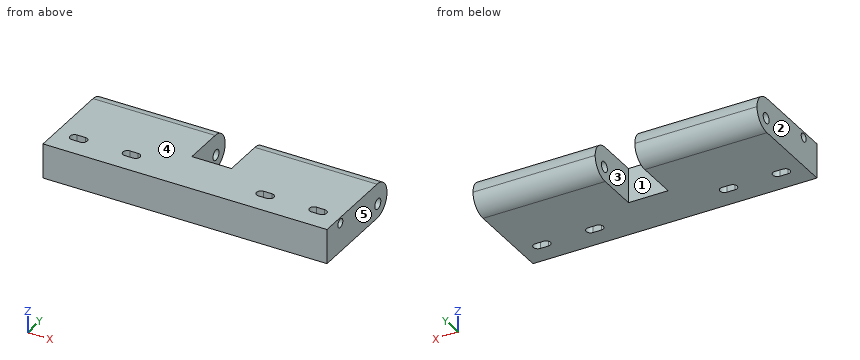
from build123d import *

# Parameters (mm, degrees)
SKETCH_1_W          = 172.02
SKETCH_1_H          = 28
EXTRUDE_1_DEPTH     = 21
SKETCH_2_W          = 74
SKETCH_2_H          = 21
EXTRUDE_2_DEPTH     = 35
CUT_EXTRUDE_1_DEPTH = 173.02
SKETCH_4_R          = 3.15
CUT_EXTRUDE_2_DEPTH = 173.02
SKETCH_6_R          = 2.6
CUT_EXTRUDE_3_DEPTH = 8
SKETCH_7_R          = 2.6
CUT_EXTRUDE_4_DEPTH = 8


with BuildPart() as part:
    # 草图1 → 凸台-拉伸1 (new body)
    with BuildSketch(Plane.XY):
        Rectangle(SKETCH_1_W, SKETCH_1_H)
        with BuildLine():
            Line((75.01, -2.7), (70.01, -2.7))
            ThreePointArc((70.01, -2.7), (67.31, 0), (70.01, 2.7))
            Line((70.01, 2.7), (75.01, 2.7))
            ThreePointArc((75.01, 2.7), (77.71, 0), (75.01, -2.7))
        make_face(mode=Mode.SUBTRACT)
        with BuildLine():
            Line((43.01, -2.7), (38.01, -2.7))
            ThreePointArc((38.01, -2.7), (35.31, 0), (38.01, 2.7))
            Line((38.01, 2.7), (43.01, 2.7))
            ThreePointArc((43.01, 2.7), (45.71, 0), (43.01, -2.7))
        make_face(mode=Mode.SUBTRACT)
        with BuildLine():
            Line((-70.01, -2.7), (-75.01, -2.7))
            ThreePointArc((-75.01, -2.7), (-77.71, 0), (-75.01, 2.7))
            Line((-75.01, 2.7), (-70.01, 2.7))
            ThreePointArc((-70.01, 2.7), (-67.31, 0), (-70.01, -2.7))
        make_face(mode=Mode.SUBTRACT)
        with BuildLine():
            Line((-43.01, 2.7), (-38.01, 2.7))
            ThreePointArc((-38.01, 2.7), (-35.31, 0), (-38.01, -2.7))
            Line((-38.01, -2.7), (-43.01, -2.7))
            ThreePointArc((-43.01, -2.7), (-45.71, 0), (-43.01, 2.7))
        make_face(mode=Mode.SUBTRACT)
    extrude(amount=EXTRUDE_1_DEPTH)

    # 草图2 → 凸台-拉伸2 (add)
    with BuildSketch(Plane(origin=(0, 14, 0), x_dir=(1, 0, 0), z_dir=(0, 1, 0))):
        with Locations((-49.01, -10.5)):
            Rectangle(SKETCH_2_W, SKETCH_2_H)
        with Locations((49.01, -10.5)):
            Rectangle(SKETCH_2_W, SKETCH_2_H)
    extrude(amount=EXTRUDE_2_DEPTH)

    # 草图3 → 切除-拉伸1 (cut, through all)
    with BuildSketch(Plane(origin=(86.01, 0, 0), x_dir=(0, 0, -1), z_dir=(1, 0, 0))):
        with BuildLine():
            Line((0, 49), (-10.5, 49))
            ThreePointArc((-10.5, 49), (-3.075378798, 45.924621202), (0, 38.5))
            Line((0, 38.5), (0, 49))
        make_face()
        with BuildLine():
            Line((-10.5, 49), (-21, 49))
            Line((-21, 49), (-21, 38.5))
            ThreePointArc((-21, 38.5), (-17.924621202, 45.924621202), (-10.5, 49))
        make_face()
    extrude(amount=-CUT_EXTRUDE_1_DEPTH, mode=Mode.SUBTRACT)

    # 草图4 → 切除-拉伸2 (cut, through all)
    with BuildSketch(Plane(origin=(86.01, 0, 0), x_dir=(0, 0, -1), z_dir=(1, 0, 0))):
        with Locations((-8.500165561, 39.35)):
            Circle(SKETCH_4_R)
    extrude(amount=-CUT_EXTRUDE_2_DEPTH, mode=Mode.SUBTRACT)

    # 草图6 → 切除-拉伸3 (cut)
    with BuildSketch(Plane(origin=(86.01, 0, 0), x_dir=(0, 0, -1), z_dir=(1, 0, 0))):
        with Locations((-17.5, 0)):
            Circle(SKETCH_6_R)
    extrude(amount=-CUT_EXTRUDE_3_DEPTH, mode=Mode.SUBTRACT)

    # 草图7 → 切除-拉伸4 (cut)
    with BuildSketch(Plane.ZY.offset(86.01)):
        with Locations((17.5, 0)):
            Circle(SKETCH_7_R)
    extrude(amount=-CUT_EXTRUDE_4_DEPTH, mode=Mode.SUBTRACT)


solid = part.part
The model under review builds one solid part; all positions refer to its coordinate system, in mm. Face numbers are marked on the shaded views. A direction names the side the tool comes from. Round coordinates to 2 decimals unless told otherwise and drop trailing zeros. Write each loop counter-clockwise with the first axis right and the second up, starting at its lowest first coordinate (ties: lowest second). Pieces come first, ordered by that corner, then holes. Notation, with made-up numbers: M -10,-34 L 30,-34 A18 ccw 30,-11 Z; hole C 69.5,16.25 d10. An arc over 180 degrees is marked long. Use a Markdown table: item, result. Add a question column.
Q1. We need section A-A, the plane y = 0. State the section outline as (x, z) points, plus the area to 3 significant figures.
Q2. To check wall thickness, follow line 1 (X direction, y = 42.5, z = 2.5); line 2 (Y direction, x = -69, z = 9); line 3 (Y direction, x = -79.5, z = 17.5). State the ranges of each line that lie inside material, in increasing order.
Q3. Insertion check: pin 1 (1 mm diameter, centred on x = 26.5, y = 41, fed in from +Z); pin 2 (7 mm diameter, centred on y = 0, z = 17.5, fed in from +X); pin 3 (6 mm diameter, centred on x = 7.5, y = 29.5, fed in from -Z); pin 4 (3 mm diameter, centred on y = 0, z = 17.5, fed in from +X). Each pin has a flat end and moves straight along its axis. Give the tip position at first contact, or say it passes through.
Q4. We need section D-D, the plane x = -62.5. State the section outline as (y, z) points, plus the area to 3 significant figures.
Q5. We need section C-C, the plane y = 20. State the section outline as (x, z) points.
Q6. We need section B-B, the plane z = 7. Count the separate pieces of the cut face and the enclosed holes in it, plus the area to 3 significant figures.
Q7. Machinability: for the marked faces 1 and 2, which of the approach directions +Z, -Z, +X, -X, +Y, -Y give a long, thin tool a straight path to every point of the face, cutting with its end or side? Answer none if there is none.
Q8. The part is to be moulded in two halves that separate along X. For the marked faces 3, 4 and 5, say which applies: pulls with the +X half, pulls with the -X half, needs draft (parallel to the pull), parting line crosses it, or undercut.
Findings below:
| question | item | result |
|---|---|---|
| 1 | outline | M -86.01,0 L -77.71,0 L -77.71,21 L -86.01,21 L -86.01,20.1 L -78.01,20.1 L -78.01,14.9 L -86.01,14.9 Z; M -67.31,0 L -45.71,0 L -45.71,21 L -67.31,21 Z; M -35.31,0 L 35.31,0 L 35.31,21 L -35.31,21 Z; M 45.71,0 L 67.31,0 L 67.31,21 L 45.71,21 Z; M 77.71,0 L 86.01,0 L 86.01,14.9 L 78.01,14.9 L 78.01,20.1 L 86.01,20.1 L 86.01,21 L 77.71,21 Z |
| 1 | area | 2,660 mm² |
| 2 | line 1 | x = -86.01 to -12.01, 12.01 to 86.01 |
| 2 | line 2 | y = -14 to -2.5, 2.5 to 36.24, 42.46 to 48.89 |
| 2 | line 3 | y = -14 to -2.6, 2.6 to 46.33 |
| 3 | pin 1 | stops at z = 20.81 |
| 3 | pin 2 | stops at x = 86.01 |
| 3 | pin 3 | passes through |
| 3 | pin 4 | stops at x = 78.01 |
| 4 | outline | M -14,0 L 38.5,0 A10.5 ccw 38.5,21 L -14,21 Z; hole C 39.35,8.5 d6.3 |
| 4 | area | 1,240 mm² |
| 5 | outline | M -86.01,0 L -12.01,0 L -12.01,21 L -86.01,21 Z; M 12.01,0 L 86.01,0 L 86.01,21 L 12.01,21 Z |
| 6 | separate pieces | 3 |
| 6 | enclosed holes | 4 |
| 6 | area | 8,890 mm² |
| 7 | face 1 | +Z, -Z, +Y |
| 7 | face 2 | +Z, -Z, -X, +Y, -Y |
| 8 | face 3 | undercut |
| 8 | face 4 | needs draft |
| 8 | face 5 | pulls with the +X half |
